from build123d import *

# Parameters (mm, degrees)
BOSS_EXTRUDE1_DEPTH = 5
SKETCH2_W           = 18
SKETCH2_H           = 24
BOSS_EXTRUDE2_DEPTH = 6
SKETCH3_R           = 2.25
CUT_EXTRUDE1_DEPTH  = 79.70196948
SKETCH4_W           = 3.5
SKETCH4_H           = 15
CUT_EXTRUDE2_DEPTH  = 79.160092119
SKETCH5_W           = 4
SKETCH5_H           = 24
BOSS_EXTRUDE3_DEPTH = 4


with BuildPart() as part:
    # Sketch1 → Boss-Extrude1 (new body)
    with BuildSketch(Plane.XY):
        with BuildLine():
            Line((-72, -12), (72, -12))
            ThreePointArc((72, -12), (74.828427125, -10.828427125), (76, -8))
            Line((76, -8), (76, 8))
            ThreePointArc((76, 8), (74.828427125, 10.828427125), (72, 12))
            Line((72, 12), (-72, 12))
            ThreePointArc((-72, 12), (-74.828427125, 10.828427125), (-76, 8))
            Line((-76, 8), (-76, -8))
            ThreePointArc((-76, -8), (-74.828427125, -10.828427125), (-72, -12))
        make_face()
    extrude(amount=BOSS_EXTRUDE1_DEPTH)

    # Sketch2 → Boss-Extrude2 (add)
    with BuildSketch(Plane.XY.offset(5)):
        with Locations((-68, 0)):
            Rectangle(SKETCH2_W, SKETCH2_H)
        with Locations((68, 0)):
            Rectangle(SKETCH2_W, SKETCH2_H)
    extrude(amount=BOSS_EXTRUDE2_DEPTH)

    # Sketch3 → Cut-Extrude1 (cut, through all)
    with BuildSketch(Plane.XY.offset(11)):
        with Locations((-68, 0)):
            Circle(SKETCH3_R)
        with Locations((68, 0)):
            Circle(SKETCH3_R)
    extrude(amount=-CUT_EXTRUDE1_DEPTH, mode=Mode.SUBTRACT)

    # Sketch4 → Cut-Extrude2 (cut, through all)
    with BuildSketch(Plane.XY.offset(5)):
        with Locations((-30, 0)):
            Rectangle(SKETCH4_W, SKETCH4_H)
        with Locations((30, 0)):
            Rectangle(SKETCH4_W, SKETCH4_H)
    extrude(amount=-CUT_EXTRUDE2_DEPTH, mode=Mode.SUBTRACT)

    # Sketch5 → Boss-Extrude3 (add)
    with BuildSketch(Plane.XY):
        with Locations((-13, 0)):
            Rectangle(SKETCH5_W, SKETCH5_H)
        with Locations((13, 0)):
            Rectangle(SKETCH5_W, SKETCH5_H)
    extrude(amount=-BOSS_EXTRUDE3_DEPTH)


solid = part.part
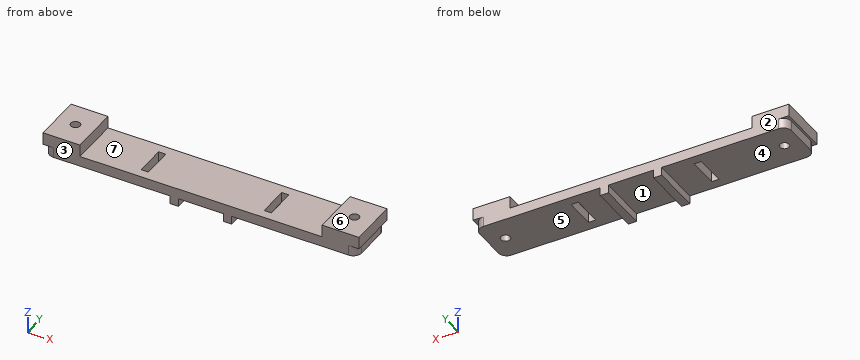
Input: part model. Units: mm. Frame: model coordinates. Face numbers are marked on the shaded views. A direction names the side the tool comes from. Coordinates: 2 decimals unless noted, no trailing zeros. Loops run counter-clockwise (first coordinate to the right, second up) from the corner with the lowest first, then second, coordinate; pieces in that order, holes last.
(1) Material intervals for probe 1 along X at (y, z) = (-0.25, 5.75); probe 2 along X at (y, z) = (6, 3); probe 3 along Y at (x, z) = (-68, 2.5), sorted ascending.
(2) Section B-B on z = 8.25. Return the cut outline in (x, y), then the cut area to 3 significant figures.
(3) Set-up query: the marked faces 3, 4, 5, 6 and 7. Return all of +Z, -Z, +X, -X, +Y, -Y with unobstructed straight access to the full face (end or side cutting, diameter ignored); none if empty.
(4) Section D-D on x = 17.5. Return the cut outline in (y, z), then the cut area to 3 significant figures.
(5) Pull-direction query (X, two-part tool) for the marked faces 1 and 2; classes: released by +X, released by -X, zero draft, split by the parting line, or undercut.
(6) Section C-C on x = 68. Return the cut outline in (y, z).
(7) Section A-A on y = -5. Return the cut outline in (x, z), then the cut area to 3 significant figures.
(8) First-contact query: pin 1 Ø1.5 at (x, y) = (-19, 1.5) entering from -Z; pin 2 Ø1.5 at (y, z) = (-2, 2) entering from -X; pin 3 Ø2 at (y, z) = (0.5, -1.5) entering from -X. Flat tips, straight axial feed; report the tip coordinate or a pass-through.
Data:
1. probe 1: x = -77 to -70.24, -65.76 to -59, 59 to 65.76, 70.24 to 77
1. probe 2: x = -76 to -31.75, -28.25 to 28.25, 31.75 to 76
1. probe 3: y = -12 to -2.25, 2.25 to 12
2. outline: (-77, -12) - (-59, -12) - (-59, 12) - (-77, 12) - close; (59, -12) - (77, -12) - (77, 12) - (59, 12) - close; hole circle Ø4.5 at (-68, 0); hole circle Ø4.5 at (68, 0)
2. area: 832 mm2
3. face 3: +Z, -Z, +X, -X, -Y
3. face 4: -Z, -X, +Y, -Y
3. face 5: -Z, +X, +Y, -Y
3. face 6: +Z, +X, -X, +Y, -Y
3. face 7: +Z, +Y, -Y
4. outline: (-12, 0) - (12, 0) - (12, 5) - (-12, 5) - close
4. area: 120 mm2
5. face 1: undercut
5. face 2: zero draft
6. outline: (-12, 0) - (-2.25, 0) - (-2.25, 11) - (-12, 11) - close; (2.25, 0) - (12, 0) - (12, 11) - (2.25, 11) - close
7. outline: (-77, 5) - (-76, 5) - (-76, 0) - (-31.75, 0) - (-31.75, 5) - (-59, 5) - (-59, 11) - (-77, 11) - close; (-28.25, 0) - (-15, 0) - (-15, -4) - (-11, -4) - (-11, 0) - (11, 0) - (11, -4) - (15, -4) - (15, 0) - (28.25, 0) - (28.25, 5) - (-28.25, 5) - close; (31.75, 0) - (76, 0) - (76, 5) - (77, 5) - (77, 11) - (59, 11) - (59, 5) - (31.75, 5) - close
7. area: 973 mm2
8. pin 1: stops at z = 0
8. pin 2: stops at x = -76
8. pin 3: stops at x = -15
